Geometry check sheet. Reference: the model listing, model coordinates, mm. A direction names the side the tool comes from. Give positions to 0.01 mm unless a question says otherwise; leave off trailing zeros. Loops run counter-clockwise (first coordinate to the right, second up) from the corner with the lowest first, then second, coordinate; pieces in that order, holes last. Notation, with made-up numbers: (-27.75, -17.5) -> (24.25, -17.5) arc R29 ccw to (24.25, 11.5) -> close; hole circle Ø2 at (2, 14.5). An arc over 180 degrees is marked (long way). Answer as a JSON object with one key per item and string values.
from build123d import *

# Parameters (mm, degrees)
F0_W     = 50.8
F0_H     = 50.8
F1_DEPTH = 50.8
F2_R     = 15.329647
F3_DEPTH = 50.8
F4_R     = 12.7
F5_DEPTH = 12.7
F6_W     = 25.4
F6_H     = 25.4
F7_DEPTH = 12.7


with BuildPart() as f1:
    # F0 (on Front) → F1 (new body)
    with BuildSketch(Plane.XZ):
        with Locations((-38.289552, 25.4)):
            Rectangle(F0_W, F0_H)
    extrude(amount=F1_DEPTH)

    # F2 (on face) → F3 (cut)
    with BuildSketch(Plane.XZ.offset(50.8)):
        with Locations((-38.289552, 25.4)):
            Circle(F2_R)
    extrude(amount=-F3_DEPTH, mode=Mode.SUBTRACT)

    # F4 (on face) → F5 (join)
    with BuildSketch(Plane.XY.offset(50.8)):
        with Locations((-38.289552, -25.4)):
            Circle(F4_R)
    extrude(amount=F5_DEPTH)

    # F6 (on face) → F7 (join)
    with BuildSketch(Plane(origin=(-63.689552, 0, 0), x_dir=(0, -1, 0), z_dir=(-1, 0, 0))):
        with Locations((25.4, 25.4)):
            Rectangle(F6_W, F6_H)
    extrude(amount=F7_DEPTH)


solid = f1.part
1) Tool access check on faces 5 (the face through (-70, -38.1, 25)), 6 (the face through (-44.3, -13.8, 50.8)), 7 (the face through (-70, -12.7, 25)). Record the directions out of +Z, -Z, +X, -X, +Y, -Y that give a thin tool (end or side, any length) a straight path to the whole face; none if there is none.
Geometry check:
{"face 5": "+Z, -Z, -X, -Y", "face 6": "+Z", "face 7": "+Z, -Z, -X, +Y"}
2) Draft check along X on faces 1 (the face through (-23.668, -25.756, 30.005)), 2 (the face through (-12.89, -25, 25)), 3 (the face through (-76.39, -25, 26)), 4 (the face through (-70, -25, 38.1)). Enter one of: pulls with the +X half, pulls with the -X half, needs draft (parallel to the pull), parting line crosses it, or undercut.
Geometry check:
{"face 1": "undercut", "face 2": "pulls with the +X half", "face 3": "pulls with the -X half", "face 4": "needs draft"}
3) Section check A-A on z = 25.4. Record the cut outline in (x, y).
Geometry check:
{"outline": "(-76.39, -38.1) -> (-63.69, -38.1) -> (-63.69, -50.8) -> (-53.62, -50.8) -> (-53.62, 0) -> (-63.69, 0) -> (-63.69, -12.7) -> (-76.39, -12.7) -> close; (-22.96, -50.8) -> (-12.89, -50.8) -> (-12.89, 0) -> (-22.96, 0) -> close"}
4) Material ranges on line 1 along X through (y, z) = (-33, 25); line 2 along Z through (x, y) = (-68.5, -24.5); line 3 along X through (y, z) = (-48, 13), recorded low to high. Write a range as from..to.
Geometry check:
{"line 1": "x = -76.39..-53.61, -22.97..-12.89", "line 2": "z = 12.7..38.1", "line 3": "x = -63.69..-47.3, -29.28..-12.89"}
5) Section check C-C on x = -39.5. Record the cut outline in (y, z), plus the area to 3 significant figures.
Geometry check:
{"outline": "(-50.8, 0) -> (0, 0) -> (0, 10.12) -> (-50.8, 10.12) -> close; (-50.8, 40.68) -> (0, 40.68) -> (0, 50.8) -> (-12.76, 50.8) -> (-12.76, 63.5) -> (-38.04, 63.5) -> (-38.04, 50.8) -> (-50.8, 50.8) -> close", "area": "1,350 mm2"}
6) Depth check by flat-ended pin: P1, Ø10, axis at x = -72.5, y = -27.5, coming from the +Z side; P2, Ø10, axis at x = -69.5, z = 20, coming from the +Y side; P3, Ø10, axis at x = -72.5, z = 24.5, coming from the -Y side. Enter the tip coordinate at first touch or a pass-through.
Geometry check:
{"P1": "stops at z = 38.1", "P2": "stops at y = -12.7", "P3": "stops at y = -38.1"}
7) Section check B-B on y = -25.4. Record the cut outline in (x, z).
Geometry check:
{"outline": "(-76.39, 12.7) -> (-63.69, 12.7) -> (-63.69, 0) -> (-12.89, 0) -> (-12.89, 50.8) -> (-25.59, 50.8) -> (-25.59, 63.5) -> (-50.99, 63.5) -> (-50.99, 50.8) -> (-63.69, 50.8) -> (-63.69, 38.1) -> (-76.39, 38.1) -> close; hole circle Ø30.66 at (-38.29, 25.4)"}
8) Section check D-D on y = -19.5. Record the cut outline in (x, z), plus the area to 3 significant figures.
Geometry check:
{"outline": "(-76.39, 12.7) -> (-63.69, 12.7) -> (-63.69, 0) -> (-12.89, 0) -> (-12.89, 50.8) -> (-27.04, 50.8) -> (-27.04, 63.5) -> (-49.54, 63.5) -> (-49.54, 50.8) -> (-63.69, 50.8) -> (-63.69, 38.1) -> (-76.39, 38.1) -> close; hole circle Ø30.66 at (-38.29, 25.4)", "area": "2,450 mm2"}
